Geometry: final body of the model. Coordinates: model frame, mm. A direction names the side the tool comes from. Give positions to 0.01 mm unless a question says otherwise; leave off trailing zeros. Write each loop counter-clockwise with the first axis right and the second up, starting at its lowest first coordinate (ties: lowest second). Pieces come first, ordered by that corner, then holes. Notation, with made-up numbers: M -9,15 L 7,15 A20 cw 7,29 Z; hole C -14,56 d6. An arc over 180 degrees is marked long. Use one line per item in the form item = value. Start each with the question number.
Item 1: Pull-direction query (X, two-part tool) for faces 1 (the cylindrical face through (74.27, 4.93, 150.19)), 2 (the flat face through (-96, 5, 158)), 3 (the cylindrical face through (0.56, 97.99, 155.15)); classes: released by +X, released by -X, zero draft, split by the parting line, or undercut.
Item 2: Section query C-C on x = 76. Return loops of the section in (y, z), then the cut area to 3 significant figures.
Item 3: Section query A-A on x = -76. Return loops of the section in (y, z).
Item 4: Section query B-B on z = 87.5. Return loops of the section in (x, y).
Item 5: Access query for faces 4 (the cylindrical face through (-1.099, 117.269, 112.476)), 5 (the flat face through (0, 38, 141)), 6 (the flat face through (-40.49, 8.38, 158.24)). Directions: +Z, -Z, +X, -X, +Y, -Y. A direction counts if a zero-diameter tool reaches every point of the face in a straight line with its end or side. Return the directions, or none.
Item 6: Material intervals for line 1 along Z through (x, y) = (-76, 5); line 2 along Z through (x, y) = (34, 51.5); line 3 along X through (y, z) = (4, 17), sorted ascending. Write a range as from..to.
Item 7: Contact query for flat-ended pins moving along their axis: P1, Ø12, axis at x = 85, z = 78, coming from the +Y side; P2, Ø3, axis at x = 18.5, y = 79, coming from the -Z side; P3, Ø17, axis at x = 13.5, z = 152, coming from the -Y side; P4, Ø14.5, axis at x = 76, z = 17, coming from the -Y side. Output: stop coordinate, or through.
Item 8: Section query D-D on y = 25. Return loops of the section in (x, z), then the cut area to 3 significant figures.
from build123d import *

# Parameters (mm, degrees)
EXTRUDE_1_DEPTH     = 34
OTHER_1_OUTLINE_R   = 8
OTHER_1_DEPTH       = 10
SKETCH_2_W          = 40
SKETCH_2_H          = 10
EXTRUDE_2_DEPTH     = 53.5
CUT_EXTRUDE_1_DEPTH = 145.890475877
FILLET_1_R          = 10
SKETCH_4_R          = 25
EXTRUDE_3_DEPTH     = 33
SKETCH_5_R          = 21
EXTRUDE_4_DEPTH     = 40
EXTRUDE_5_DEPTH     = 10


# Read off the part's stored shape, not the designer's step: Полость1
with BuildPart() as part:
    # Эскиз1 → Бобышка-Вытянуть1 (new body)
    with BuildSketch(Plane.XY):
        Polygon((96, 0), (51, 0), (29.67790849, 17), (0, 17), (0, 101), (40, 101), (40, 21.559615382), (54.498539822, 10), (96, 10), align=None)
    extrude(amount=EXTRUDE_1_DEPTH)

    # Полость1 outline → Полость1 (cut)
    with BuildSketch(Plane(origin=(0, 0, 0), x_dir=(1, 0, 0), z_dir=(0, 1, 0))):
        with Locations((76, -17)):
            Circle(OTHER_1_OUTLINE_R)
    extrude(amount=OTHER_1_DEPTH, mode=Mode.SUBTRACT)

    # Эскиз2 → Бобышка-Вытянуть2 (add)
    with BuildSketch(Plane.XY.offset(34)):
        with Locations((20, 96)):
            Rectangle(SKETCH_2_W, SKETCH_2_H)
    extrude(amount=EXTRUDE_2_DEPTH)

    # Эскиз3 → Вырез-Вытянуть1 (cut, through all)
    with BuildSketch(Plane(origin=(40, 0, 0), x_dir=(0, 0, -1), z_dir=(1, 0, 0))):
        Polygon((0, 101), (-17, 101), (-17, 38.559615382), (0, 21.559615382), align=None)
    extrude(amount=-CUT_EXTRUDE_1_DEPTH, mode=Mode.SUBTRACT)

    # Скругление1
    fillet_1_edges = [part.edges().sort_by_distance(p)[0] for p in [
        (20, 91, 34),
        (20, 38.559615382, 17),
        (20, 101, 17),
    ]]
    fillet(fillet_1_edges, radius=FILLET_1_R)

    # Зеркальное отражение1: part across plane


with BuildPart() as part_1:
    add(part.part)
    add(part.part.mirror(Plane(origin=(0, 17, 173.344895852), x_dir=(0, 0, 1), z_dir=(1, 0, 0))))

    # Зеркальное отражение2: part across plane


with BuildPart() as part_2:
    add(part_1.part)
    add(part_1.part.mirror(Plane(origin=(0, -14, 87.5), x_dir=(1, 0, 0), z_dir=(0, 0, 1))))

    # Эскиз4 → Бобышка-Вытянуть3 (add)
    with BuildSketch(Plane(origin=(0, 101, 0), x_dir=(1, 0, 0), z_dir=(0, 1, 0))):
        with Locations(Location((0, -87.5, 0), (0, 0, 90))):
            Circle(SKETCH_4_R)
    extrude(amount=EXTRUDE_3_DEPTH)

    # Эскиз5 → Бобышка-Вытянуть4 (add)
    with BuildSketch(Plane(origin=(0, 134, 0), x_dir=(1, 0, 0), z_dir=(0, 1, 0))):
        with Locations(Location((0, -87.5, 0), (0, 0, 180))):
            Circle(SKETCH_5_R)
    extrude(amount=EXTRUDE_4_DEPTH)

    # Эскиз6 → Бобышка-Вытянуть5 (add)
    with BuildSketch(Plane(origin=(0, 101, 0), x_dir=(1, 0, 0), z_dir=(0, 1, 0))):
        Polygon((131.15, -108.65), (136.15, -103.65), (136.15, -71.35), (131.15, -66.35), (40, -27), (40, -148), align=None)
    extrude(amount=-EXTRUDE_5_DEPTH)


solid = part_2.part
Answer sheet:
q1.face_1 = undercut
q1.face_2 = released by -X
q1.face_3 = zero draft
q2.outline = M 0,0 L 10,0 L 10,9 L 0,9 Z; M 0,25 L 10,25 L 10,34 L 0,34 Z; M 0,141 L 10,141 L 10,150 L 0,150 Z; M 0,166 L 10,166 L 10,175 L 0,175 Z; M 91,42.54 L 101,42.54 L 101,132.46 L 91,132.46 Z
q2.area = 1,260 mm2
q3.outline = M 0,0 L 10,0 L 10,9 L 0,9 Z; M 0,25 L 10,25 L 10,34 L 0,34 Z; M 0,141 L 10,141 L 10,150 L 0,150 Z; M 0,166 L 10,166 L 10,175 L 0,175 Z
q4.outline = M -40,91 L 136.15,91 L 136.15,101 L 25,101 L 25,134 L 21,134 L 21,174 L -21,174 L -21,134 L -25,134 L -25,101 L -40,101 Z
q5.face_4 = +Y
q5.face_5 = +X, -X, -Y
q5.face_6 = +Z, -Z, -Y
q6.line_1 = 0..9, 25..34, 141..150, 166..175
q6.line_2 = 17..34, 141..158
q6.line_3 = -96..-84, -68..-45.98, 45.98..68, 84..96
q7.P1 = 101
q7.P2 = 17
q7.P3 = 17
q7.P4 = through
q8.outline = M -40,3.44 L 40,3.44 L 40,34 L -40,34 Z; M -40,141 L 40,141 L 40,171.56 L -40,171.56 Z
q8.area = 4,890 mm2
